Could you check a few things on this model? Use its own coordinates, in mm. A direction names the side the tool comes from. Coordinates: 2 decimals unless noted, no trailing zeros. Loops run counter-clockwise (first coordinate to the right, second up) from the corner with the lowest first, then second, coordinate; pieces in that order, holes last.
from build123d import *

# Parameters (mm, degrees)
F0_R     = 3.175
F1_DEPTH = 2
F2_R     = 6.5
F3_DEPTH = 2
F4_R     = 3
F5_DEPTH = 1
F6_R     = 1.5
F7_DEPTH = 25
F8_R     = 4.15
F8_R_2   = 3.175
F9_DEPTH = 1


with BuildPart() as f1:
    # F0 (on Top) → F1 (new body)
    with BuildSketch(Plane.XY):
        Circle(F0_R)
    extrude(amount=F1_DEPTH)

    # F2 (on face) → F3 (join)
    with BuildSketch(Plane.XY.offset(2)):
        Circle(F2_R)
    extrude(amount=F3_DEPTH)

    # F4 (on face) → F5 (cut)
    with BuildSketch(Plane.XY.offset(4)):
        Circle(F4_R)
    extrude(amount=-F5_DEPTH, mode=Mode.SUBTRACT)

    # F6 (on face) → F7 (cut)
    with BuildSketch(Plane(origin=(0, 0, 0), x_dir=(1, 0, 0), z_dir=(0, 0, -1))):
        Circle(F6_R)
    extrude(amount=-F7_DEPTH, mode=Mode.SUBTRACT)

    # F8 (on face) → F9 (join)
    with BuildSketch(Plane(origin=(0, 0, 2), x_dir=(1, 0, 0), z_dir=(0, 0, -1))):
        Circle(F8_R)
        Circle(F8_R_2, mode=Mode.SUBTRACT)
    extrude(amount=F9_DEPTH)


solid = f1.part
1) Imagine slicing it at C-C on z = 1.8. List the corners of the cut face in (x, y) for me, plus the area to 3 significant figures.
2) For faces 4 (the cylindrical face through (-3, 0.1, 3.5)), 5 (the cylindrical face through (-0.69, -3.1, 0.49)), 6 (the cylindrical face through (-5.158, -3.955, 2.986)), which set-ups out of +Z, -Z, +X, -X, +Y, -Y let a thin tool reach every point of the face, with its end or its side?
3) Imagine slicing it at D-D on y = -2.75. List the corners of the cut face in (x, z) for me.
4) If I drill on L1, parallel to X at y = 0, z = 1.85; L2, parallel to Y at x = 0, z = 3.55, over which ranges is the centre line in solid material (lowest first)?
5) Will these pins go through, and if not, where does the flat tip stop? pin 1 (3.5 mm diameter, centred on x = 0, y = 0, fed in from +Z); pin 2 (2 mm diameter, centred on y = -3.5, z = 2.5, fed in from +X).
6) Imagine slicing it at A-A on y = 0. List the corners of the cut face in (x, z) for me (3 decimals).
7) We'd pull the mould along X, two halves only. Please class faces 1 (the flat face through (1.3, -1.3, 3)), 2 (the cylindrical face through (-0.9, 4.05, 1.51)), 3 (the flat face through (3, -1, 4)): released by +X, released by -X, zero draft, split by the parting line, or undercut.
Solved:
1. outline: circle Ø8.3 at (0, 0); hole circle Ø3 at (0, 0)
1. area: 47.0 mm2
2. face 4: +Z
2. face 5: -Z
2. face 6: +Z, -Z
3. outline: (-5.89, 2) - (-3.11, 2) - (-3.11, 1) - (-1.59, 1) - (-1.59, 0) - (1.59, 0) - (1.59, 1) - (3.11, 1) - (3.11, 2) - (5.89, 2) - (5.89, 4) - (1.2, 4) - (1.2, 3) - (-1.2, 3) - (-1.2, 4) - (-5.89, 4) - close
4. L1: x = -4.15 to -1.5, 1.5 to 4.15
4. L2: y = -6.5 to -3, 3 to 6.5
5. pin 1: stops at z = 3
5. pin 2: stops at x = 6
6. outline: (-6.5, 2) - (-4.15, 2) - (-4.15, 1) - (-3.175, 1) - (-3.175, 0) - (-1.5, 0) - (-1.5, 3) - (-3, 3) - (-3, 4) - (-6.5, 4) - close; (1.5, 0) - (3.175, 0) - (3.175, 1) - (4.15, 1) - (4.15, 2) - (6.5, 2) - (6.5, 4) - (3, 4) - (3, 3) - (1.5, 3) - close
7. face 1: undercut
7. face 2: split by the parting line
7. face 3: zero draft
